Geometry check sheet. Reference: the model listing, model coordinates, mm. Face numbers are marked on the shaded views. A direction names the side the tool comes from. Coordinates: 2 decimals unless noted, no trailing zeros. Order: outer loops, then holes, each group sorted by start corner. A loop starts at its lowest first (then second) coordinate and runs counter-clockwise, first axis right, second up. Notation, with made-up numbers: (6, 73.25) - (58, 73.25) arc R16 cw to (58, 93.25) - close; hole circle Ø3 at (8, -21). An arc over 180 degrees is marked (long way). Return JSON: item names as keys, results as strings. Group by question number.
Item 1: Tool access check on the marked faces 1 and 2. Record the directions out of +Z, -Z, +X, -X, +Y, -Y that give a thin tool (end or side, any length) a straight path to the whole face; none if there is none.
Item 2: Section check C-C on y = 6.5. Enter the section's corners in (x, z), then the cut area to 3 significant figures.
Item 3: Scan lines: probe 1 along Z at (x, y) = (-5.5, -3.75); probe 2 along Z at (x, y) = (-4.25, -4); probe 3 along Y at (x, z) = (0, 0.25). Record each from-to range of solid material in increasing order.
Item 4: Section check D-D on x = 6.75. Enter the section's corners in (y, z), then the cut area to 3 significant figures.
Item 5: Gauge pin test, flat ends, axial feed: pin 1 (2 mm diameter, centred on x = 3, z = -5.5, fed in from +Y); pin 2 (8 mm diameter, centred on y = 0, z = -5, fed in from -X); pin 3 (1.5 mm diameter, centred on x = 0, z = 1.5, fed in from -Y); pin 4 (3 mm diameter, centred on x = 0, y = 0, fed in from -Z). Record the tip position at first contact, or that the pin passes through.
Item 6: Draft check along Z on the marked faces 3, 4, 5 and 6. Enter one of: pulls with the +Z half, pulls with the -Z half, needs draft (parallel to the pull), parting line crosses it, or undercut.
Item 7: Section check A-A on y = 0. Enter the section's corners in (x, z), then the cut area to 3 significant figures.
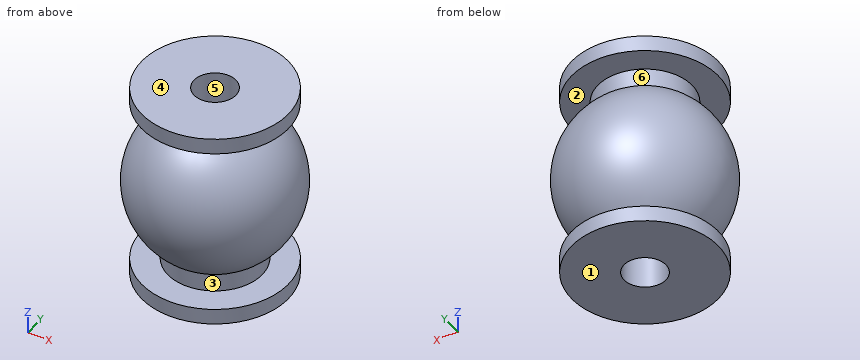
from build123d import *

# Parameters (mm, degrees)
F_4_0_4_DIAMETER_HOLE1_D = 4


with BuildPart() as part:
    # Sketch1 → Revolve1 (revolve)
    with BuildSketch(Plane(origin=(0, 0, 0), x_dir=(1, 0, 0), z_dir=(0, 1, 0))):
        with BuildLine():
            Line((-4.5, -6.309714732), (-4.5, -8))
            Line((-4.5, -8), (-7, -8))
            Line((-7, -8), (-7, -9.5))
            Line((-7, -9.5), (0, -9.5))
            Line((0, -9.5), (0, 9.5))
            Line((0, 9.5), (-7, 9.5))
            Line((-7, 9.5), (-7, 8))
            Line((-7, 8), (-4.5, 8))
            Line((-4.5, 8), (-4.5, 6.309714732))
            ThreePointArc((-4.5, 6.309714732), (-7.75, 0), (-4.5, -6.309714732))
        make_face()
    revolve(axis=Axis((0, 0, 9.5), (0, 0, -1)))

    # Ø4.0 (4) Diameter Hole1 (through all)
    with Locations(Plane.XY.offset(9.5)):
        with Locations((0, 0)):
            Hole(F_4_0_4_DIAMETER_HOLE1_D / 2)


solid = part.part
Computed:
{
 "1": {"face 1": "-Z, +X, -X, +Y, -Y", "face 2": "none"},
 "2": {"outline": "circle Ø8.44 at (0, 0); (-2.6, -9.5) - (2.6, -9.5) - (2.6, -8) - (-2.6, -8) - close; (-2.6, 8) - (2.6, 8) - (2.6, 9.5) - (-2.6, 9.5) - close", "area": "71.5 mm²"},
 "3": {"probe 1": "z = -9.5 to -8, -3.97 to 3.97, 8 to 9.5", "probe 2": "z = -9.5 to -8, -5.1 to 5.1, 8 to 9.5", "probe 3": "y = -7.75 to -2, 2 to 7.75"},
 "4": {"outline": "circle Ø7.62 at (0, 0); (-1.85, -9.5) - (1.85, -9.5) - (1.85, -8) - (-1.85, -8) - close; (-1.85, 8) - (1.85, 8) - (1.85, 9.5) - (-1.85, 9.5) - close", "area": "56.7 mm²"},
 "5": {"pin 1": "stops at y = 5.69", "pin 2": "stops at x = -7.69", "pin 3": "stops at y = -7.71", "pin 4": "passes through"},
 "6": {"face 3": "undercut", "face 4": "pulls with the +Z half", "face 5": "needs draft", "face 6": "undercut"},
 "7": {"outline": "(-7, -9.5) - (-2, -9.5) - (-2, 9.5) - (-7, 9.5) - (-7, 8) - (-4.5, 8) - (-4.5, 6.31) arc R7.75 ccw to (-4.5, -6.31) - (-4.5, -8) - (-7, -8) - close; (2, -9.5) - (7, -9.5) - (7, -8) - (4.5, -8) - (4.5, -6.31) arc R7.75 ccw to (4.5, 6.31) - (4.5, 8) - (7, 8) - (7, 9.5) - (2, 9.5) - close", "area": "167 mm²"}
}
